Verification items for the finished model (mm, model axes). A direction names the side the tool comes from. Round coordinates to 2 decimals unless told otherwise and drop trailing zeros. Write each loop counter-clockwise with the first axis right and the second up, starting at its lowest first coordinate (ties: lowest second). Pieces come first, ordered by that corner, then holes. Notation, with made-up numbers: (-10.75, 61) -> (30.25, 61) arc R20 ccw to (30.25, 87) -> close; hole circle Ø1 at (30.5, 65). An arc over 180 degrees is marked (long way). Answer as a JSON object with one key per item and string values. Group by question number.
(1) Set-up check for faces 5 (the face through (-108.294, -2, 55)), 6 (the face through (-71, -2, 6.335)), 7 (the face through (-106, -2, 67.549)), 8 (the face through (-15.324, -2.004, 58.698)), 9 (the face through (-10, -2, 10.399)): record each of +Z, -Z, +X, -X, +Y, -Y from which the full face is reachable in a straight line by a thin tool's end or side.
(2) Sectioned sample at D-D on y = -1.35. Count the separate pieces of the cut face and the enclosed holes in it, and give its area (3 significant figures).
(3) Sectioned sample at A-A on z = 65. Record the cut outline in (x, y).
(4) Gauge pin test, flat ends, axial feed: pin 1 Ø2 at (x, y) = (-53.5, -1) entering from -Z; pin 2 Ø1.5 at (y, z) = (-3, 80) entering from +X; pin 3 Ø1.2 at (x, y) = (-23, -2) entering from +Z. Record the tip position at first contact, or that the pin passes through.
(5) Sectioned sample at B-B on z = 85. Record the cut outline in (x, y), and give its area (3 significant figures).
(6) Draft check along Z on faces 1 (the face through (-67.002, -2.004, 24.249)), 2 (the face through (-83.317, -2, 8)), 3 (the face through (-55, -2, 10.399)), 4 (the face through (-63.585, -2.004, 74.007)). Enter one of: released by +Z, released by -Z, zero draft, split by the parting line, or undercut.
(7) Sectioned sample at C-C on x = -95. Record the cut outline in (y, z), and give its area (3 significant figures).
(8) Scan lines: L1, parallel to Z at x = -63.5, y = -2.85; L2, parallel to X at y = -3.15, z = 68; L3, parallel to X at y = -1.9, z = 56. Record each from-to range of solid material in increasing order. Write a range as from..to.
```python
from build123d import *

# Parameters (mm, degrees)
F0_R     = 1.5367
F1_DEPTH = 4.064


with BuildPart() as f1:
    # F0 (on Front) → F1 (new body)
    with BuildSketch(Plane.XZ):
        with BuildLine():
            Line((-104.230369, 34.021411), (-104.230369, 10.399411))
            Line((-104.230369, 10.399411), (-83.317001, 10.399411))
            Line((-83.317001, 10.399411), (-83.317001, 6.335411))
            Line((-83.317001, 6.335411), (-57.917001, 6.335411))
            Line((-57.917001, 6.335411), (-57.917001, 10.399411))
            Line((-57.917001, 10.399411), (-51.567001, 10.399411))
            ThreePointArc((-51.567001, 10.399411), (-50.286289, 23.155259), (-44.800168, 34.742078))
            ThreePointArc((-44.800168, 34.742078), (-39.353114, 39.16509), (-32.517001, 40.746542))
            Line((-32.517001, 40.746542), (-32.517001, 50.34544))
            Line((-32.517001, 50.34544), (-32.517001, 86.599411))
            Line((-32.517001, 86.599411), (-57.917001, 86.599411))
            Line((-57.917001, 86.599411), (-57.917001, 90.663411))
            Line((-57.917001, 90.663411), (-83.317001, 90.663411))
            Line((-83.317001, 90.663411), (-83.317001, 86.599411))
            Line((-83.317001, 86.599411), (-104.230369, 86.599411))
            Line((-104.230369, 86.599411), (-104.230369, 67.549411))
            Line((-104.230369, 67.549411), (-108.294369, 67.549411))
            Line((-108.294369, 67.549411), (-108.294369, 64.219405))
            Line((-108.294369, 64.219405), (-108.294369, 42.149411))
            Line((-108.294369, 42.149411), (-104.230369, 42.149411))
            Line((-104.230369, 42.149411), (-104.230369, 34.021411))
        make_face()
        with Locations((-65.78223, 25.183681)):
            Circle(F0_R, mode=Mode.SUBTRACT)
        with Locations((-89.67876, 51.61067)):
            Circle(F0_R, mode=Mode.SUBTRACT)
        with BuildLine():
            ThreePointArc((-58.96075, 66.41181), (-50.670405, 60.208094), (-47.516996, 50.34544))
            ThreePointArc((-47.516996, 50.34544), (-47.59417, 48.72743), (-47.824991, 47.124109))
            Line((-47.824991, 47.124109), (-46.479494, 46.347286))
            ThreePointArc((-46.479494, 46.347286), (-45.915131, 45.241108), (-46.151868, 44.022055))
            Line((-46.151868, 44.022055), (-49.858222, 37.602462))
            ThreePointArc((-49.858222, 37.602462), (-50.795585, 36.787915), (-52.035744, 36.723579))
            Line((-52.035744, 36.723579), (-53.381241, 37.500402))
            ThreePointArc((-53.381241, 37.500402), (-64.517, 33.345436), (-75.652759, 37.500402))
            Line((-75.652759, 37.500402), (-76.998257, 36.723579))
            ThreePointArc((-76.998257, 36.723579), (-78.238416, 36.787915), (-79.175778, 37.602462))
            Line((-79.175778, 37.602462), (-82.882132, 44.022055))
            ThreePointArc((-82.882132, 44.022055), (-83.118869, 45.241108), (-82.554507, 46.347286))
            Line((-82.554507, 46.347286), (-81.209009, 47.124109))
            ThreePointArc((-81.209009, 47.124109), (-79.239436, 58.845442), (-70.07325, 66.41181))
            Line((-70.07325, 66.41181), (-70.07325, 67.965456))
            ThreePointArc((-70.07325, 67.965456), (-69.397453, 69.007298), (-68.223354, 69.411804))
            Line((-68.223354, 69.411804), (-60.810646, 69.411804))
            ThreePointArc((-60.810646, 69.411804), (-59.636547, 69.007298), (-58.96075, 67.965456))
            Line((-58.96075, 67.965456), (-58.96075, 66.41181))
        make_face(mode=Mode.SUBTRACT)
        with BuildLine():
            ThreePointArc((-40.227387, 50.34544), (-39.35524, 50.61691), (-38.483094, 50.34544))
            ThreePointArc((-38.483094, 50.34544), (-37.994786, 49.79478), (-37.81854, 49.08021))
            ThreePointArc((-37.81854, 49.08021), (-40.06981, 47.719756), (-40.227387, 50.34544))
        make_face(mode=Mode.SUBTRACT)
        with Locations((-63.25177, 75.5072)):
            Circle(F0_R, mode=Mode.SUBTRACT)
        with BuildLine():
            Line((-32.517001, 50.34544), (-32.517001, 40.746542))
            ThreePointArc((-32.517001, 40.746542), (-25.680887, 39.16509), (-20.233833, 34.742078))
            ThreePointArc((-20.233833, 34.742078), (-14.747713, 23.155259), (-13.467001, 10.399411))
            Line((-13.467001, 10.399411), (-13.044369, 10.399411))
            Line((-13.044369, 10.399411), (-7.117001, 10.399411))
            Line((-7.117001, 10.399411), (-7.117001, 6.335411))
            Line((-7.117001, 6.335411), (18.282999, 6.335411))
            Line((18.282999, 6.335411), (18.282999, 10.399411))
            Line((18.282999, 10.399411), (40.041631, 10.399411))
            Line((40.041631, 10.399411), (40.041631, 34.021411))
            Line((40.041631, 34.021411), (40.041631, 42.149411))
            Line((40.041631, 42.149411), (43.260368, 42.149411))
            Line((43.260368, 42.149411), (43.260368, 67.549411))
            Line((43.260368, 67.549411), (40.041631, 67.549411))
            Line((40.041631, 67.549411), (40.041631, 86.599411))
            Line((40.041631, 86.599411), (18.282999, 86.599411))
            Line((18.282999, 86.599411), (18.282999, 90.663411))
            Line((18.282999, 90.663411), (-7.117001, 90.663411))
            Line((-7.117001, 90.663411), (-7.117001, 86.599411))
            Line((-7.117001, 86.599411), (-32.517001, 86.599411))
            Line((-32.517001, 86.599411), (-32.517001, 50.34544))
        make_face()
        with Locations((0.748229, 25.183681)):
            Circle(F0_R, mode=Mode.SUBTRACT)
        with Locations((-25.678761, 49.08021)):
            Circle(F0_R, mode=Mode.SUBTRACT)
        with BuildLine():
            Line((5.039249, 67.965456), (5.039249, 66.41181))
            ThreePointArc((5.039249, 66.41181), (14.205434, 58.845442), (16.175008, 47.124109))
            Line((16.175008, 47.124109), (17.520505, 46.347286))
            ThreePointArc((17.520505, 46.347286), (18.084868, 45.241108), (17.848131, 44.022055))
            Line((17.848131, 44.022055), (14.141777, 37.602462))
            ThreePointArc((14.141777, 37.602462), (13.204414, 36.787915), (11.964255, 36.723579))
            Line((11.964255, 36.723579), (10.618758, 37.500402))
            ThreePointArc((10.618758, 37.500402), (-0.517001, 33.345436), (-11.65276, 37.500402))
            Line((-11.65276, 37.500402), (-12.998258, 36.723579))
            ThreePointArc((-12.998258, 36.723579), (-14.238417, 36.787915), (-15.175779, 37.602462))
            Line((-15.175779, 37.602462), (-18.882133, 44.022055))
            ThreePointArc((-18.882133, 44.022055), (-19.11887, 45.241108), (-18.554508, 46.347286))
            Line((-18.554508, 46.347286), (-17.20901, 47.124109))
            ThreePointArc((-17.20901, 47.124109), (-15.239437, 58.845442), (-6.073251, 66.41181))
            Line((-6.073251, 66.41181), (-6.073251, 67.965456))
            ThreePointArc((-6.073251, 67.965456), (-5.397454, 69.007298), (-4.223355, 69.411804))
            Line((-4.223355, 69.411804), (3.189353, 69.411804))
            ThreePointArc((3.189353, 69.411804), (4.363452, 69.007298), (5.039249, 67.965456))
        make_face(mode=Mode.SUBTRACT)
        with Locations((24.644759, 51.61067)):
            Circle(F0_R, mode=Mode.SUBTRACT)
        with BuildLine():
            ThreePointArc((-1.782231, 73.9705), (-2.868842, 76.593811), (-0.245531, 75.5072))
            ThreePointArc((-0.245531, 75.5072), (-0.69562, 74.420589), (-1.782231, 73.9705))
        make_face(mode=Mode.SUBTRACT)
    extrude(amount=F1_DEPTH)


solid = f1.part
```
Computed values:
{
 "1": {"face 5": "+Z, -Z, -X, +Y, -Y", "face 6": "-Z, +X, -X, +Y, -Y", "face 7": "+Z, -X, +Y, -Y", "face 8": "+Y, -Y", "face 9": "-Z, +Y, -Y"},
 "2": {"separate pieces": "1", "enclosed holes": "10", "area": "8,630 mm2"},
 "3": {"outline": "(-108.29, -4.06) -> (-73.13, -4.06) -> (-73.13, 0) -> (-108.29, 0) -> close; (-55.9, -4.06) -> (-9.13, -4.06) -> (-9.13, 0) -> (-55.9, 0) -> close; (8.1, -4.06) -> (43.26, -4.06) -> (43.26, 0) -> (8.1, 0) -> close"},
 "4": {"pin 1": "z = 10.4", "pin 2": "x = 40.04", "pin 3": "z = 86.6"},
 "5": {"outline": "(-104.23, -4.06) -> (40.04, -4.06) -> (40.04, 0) -> (-104.23, 0) -> close", "area": "586 mm2"},
 "6": {"face 1": "undercut", "face 2": "zero draft", "face 3": "released by -Z", "face 4": "undercut"},
 "7": {"outline": "(-4.06, 10.4) -> (0, 10.4) -> (0, 86.6) -> (-4.06, 86.6) -> close", "area": "310 mm2"},
 "8": {"L1": "6.34..33.38, 69.41..73.99, 77.02..90.66", "L2": "-104.23..-70.06, -58.97..-6.06, 5.03..40.04", "L3": "-108.29..-80.55, -48.48..-16.55, 15.52..43.26"}
}
